CAD build for the part. Positions are in the model's coordinates, mm. Face numbers are marked on the shaded views. Coordinates: 2 decimals unless noted, no trailing zeros. Order: outer loops, then holes, each group sorted by start corner. A loop starts at its lowest first (then second) coordinate and runs counter-clockwise, first axis right, second up. Notation, with made-up numbers: (35, -32) - (79, -32) arc R32 cw to (79, -1) - close; hole circle Ø7 at (-16, 33.25). An arc over 180 degrees is marked (long way). Use one line per item in the form item = value.
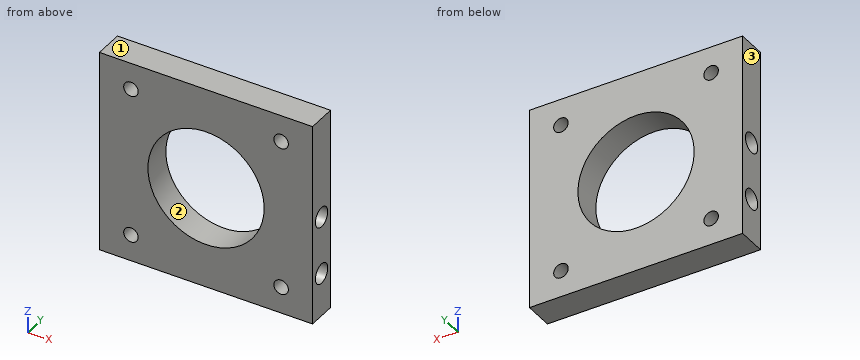
```python
from build123d import *

# Parameters (mm, degrees)
SKETCH1_W           = 44
SKETCH1_H           = 6
BOSS_EXTRUDE1_DEPTH = 42
CUT_EXTRUDE4_REACH  = 8
SKETCH5_R           = 12
SKETCH5_R_2         = 1.5
SKETCH6_R           = 2.05
CUT_EXTRUDE5_DEPTH  = 6
SKETCH7_R           = 2.05
CUT_EXTRUDE6_DEPTH  = 6


with BuildPart() as part:
    # Sketch1 → Boss-Extrude1 (new body)
    with BuildSketch(Plane.XY):
        Rectangle(SKETCH1_W, SKETCH1_H)
    extrude(amount=BOSS_EXTRUDE1_DEPTH)

    # Sketch5 → Cut-Extrude4 (cut, up to next)
    with BuildSketch(Plane(origin=(0, 3, 0), x_dir=(1, 0, 0), z_dir=(0, 1, 0)), mode=Mode.PRIVATE) as cut_extrude4_sk1:
        with Locations((0, -21)):
            Circle(SKETCH5_R)
    cut_extrude4_tool1 = extrude(cut_extrude4_sk1.sketch, amount=-CUT_EXTRUDE4_REACH, mode=Mode.PRIVATE) & part.part
    add(cut_extrude4_tool1.solids().sort_by_distance((0, 3, 21))[0], mode=Mode.SUBTRACT)
    # Sketch5 → Cut-Extrude4 (cut, up to next)
    with BuildSketch(Plane(origin=(0, 3, 0), x_dir=(1, 0, 0), z_dir=(0, 1, 0)), mode=Mode.PRIVATE) as cut_extrude4_sk2:
        with Locations((-15.5, -5.5)):
            Circle(SKETCH5_R_2)
    cut_extrude4_tool2 = extrude(cut_extrude4_sk2.sketch, amount=-CUT_EXTRUDE4_REACH, mode=Mode.PRIVATE) & part.part
    add(cut_extrude4_tool2.solids().sort_by_distance((-15.5, 3, 5.5))[0], mode=Mode.SUBTRACT)
    # Sketch5 → Cut-Extrude4 (cut, up to next)
    with BuildSketch(Plane(origin=(0, 3, 0), x_dir=(1, 0, 0), z_dir=(0, 1, 0)), mode=Mode.PRIVATE) as cut_extrude4_sk3:
        with Locations((15.5, -5.5)):
            Circle(SKETCH5_R_2)
    cut_extrude4_tool3 = extrude(cut_extrude4_sk3.sketch, amount=-CUT_EXTRUDE4_REACH, mode=Mode.PRIVATE) & part.part
    add(cut_extrude4_tool3.solids().sort_by_distance((15.5, 3, 5.5))[0], mode=Mode.SUBTRACT)
    # Sketch5 → Cut-Extrude4 (cut, up to next)
    with BuildSketch(Plane(origin=(0, 3, 0), x_dir=(1, 0, 0), z_dir=(0, 1, 0)), mode=Mode.PRIVATE) as cut_extrude4_sk4:
        with Locations((15.5, -36.5)):
            Circle(SKETCH5_R_2)
    cut_extrude4_tool4 = extrude(cut_extrude4_sk4.sketch, amount=-CUT_EXTRUDE4_REACH, mode=Mode.PRIVATE) & part.part
    add(cut_extrude4_tool4.solids().sort_by_distance((15.5, 3, 36.5))[0], mode=Mode.SUBTRACT)
    # Sketch5 → Cut-Extrude4 (cut, up to next)
    with BuildSketch(Plane(origin=(0, 3, 0), x_dir=(1, 0, 0), z_dir=(0, 1, 0)), mode=Mode.PRIVATE) as cut_extrude4_sk5:
        with Locations((-15.5, -36.5)):
            Circle(SKETCH5_R_2)
    cut_extrude4_tool5 = extrude(cut_extrude4_sk5.sketch, amount=-CUT_EXTRUDE4_REACH, mode=Mode.PRIVATE) & part.part
    add(cut_extrude4_tool5.solids().sort_by_distance((-15.5, 3, 36.5))[0], mode=Mode.SUBTRACT)

    # Sketch6 → Cut-Extrude5 (cut)
    with BuildSketch(Plane.ZY.offset(22)):
        with Locations((9, 0)):
            Circle(SKETCH6_R)
        with Locations((21, 0)):
            Circle(SKETCH6_R)
    extrude(amount=-CUT_EXTRUDE5_DEPTH, mode=Mode.SUBTRACT)

    # Sketch7 → Cut-Extrude6 (cut)
    with BuildSketch(Plane(origin=(22, 0, 0), x_dir=(0, 0, -1), z_dir=(1, 0, 0))):
        with Locations((-9, 0)):
            Circle(SKETCH7_R)
        with Locations((-21, 0)):
            Circle(SKETCH7_R)
    extrude(amount=-CUT_EXTRUDE6_DEPTH, mode=Mode.SUBTRACT)


solid = part.part
```
Item 1: Drop flat-ended pins along their axis: pin 1 (1.8 mm diameter, centred on x = -15.5, z = 5.5, fed in from +Y); pin 2 (2 mm diameter, centred on y = 0.5, z = 21, fed in from +X); pin 3 (2 mm diameter, centred on y = 0.5, z = 21, fed in from -X). Give the stop position or say it passes through.
Derived:
pin_1 = through
pin_2 = 16
pin_3 = -16
Item 2: Cut at D-D, the plane z = 29. Write the cut outline in (x, y).
Derived:
outline = (-22, -3) - (-8.94, -3) - (-8.94, 3) - (-22, 3) - close; (8.94, -3) - (22, -3) - (22, 3) - (8.94, 3) - close
Item 3: Cut at A-A, the plane z = 5.5. Write the cut outline in (x, y), plus the area to 3 significant figures.
Derived:
outline = (-22, -3) - (-17, -3) - (-17, 3) - (-22, 3) - close; (-14, -3) - (14, -3) - (14, 3) - (-14, 3) - close; (17, -3) - (22, -3) - (22, 3) - (17, 3) - close
area = 228 mm²
Item 4: Two-plate mould, pull along Z, no slides. Class the marked faces 1, 2 and 3: +Z half, -Z half, draft (parallel to the pull), parting line (faces both ways), or undercut.
Derived:
face_1 = +Z half
face_2 = undercut
face_3 = draft
Item 5: Cut at C-C, the plane x = 15.5. Write the cut outline in (y, z), plus the area to 3 significant figures.
Derived:
outline = (-3, 0) - (3, 0) - (3, 4) - (-3, 4) - close; (-3, 7) - (3, 7) - (3, 35) - (-3, 35) - close; (-3, 38) - (3, 38) - (3, 42) - (-3, 42) - close
area = 216 mm²
Item 6: Drill centre lines: line 1 (X direction, y = -0.05, z = 5.5); line 2 (Z direction, x = 15.5, y = -1.15); line 3 (Z direction, x = 0, y = 0.2). Where is each one in solid material? Low to high. Write a range as [from, to].
Derived:
line_1 = [-22, -17], [-14, 14], [17, 22]
line_2 = [0, 4], [7, 35], [38, 42]
line_3 = [0, 9], [33, 42]
Item 7: Cut at B-B, the plane x = 0. Write the cut outline in (y, z).
Derived:
outline = (-3, 0) - (3, 0) - (3, 9) - (-3, 9) - close; (-3, 33) - (3, 33) - (3, 42) - (-3, 42) - close
